from build123d import *

# Parameters (mm, degrees)
BOSS_EXTRUDE1_DEPTH      = 170
SKETCH7_W                = 5
SKETCH7_H                = 142.5
BOSS_EXTRUDE2_DEPTH      = 130
SKETCH9_W                = 160
SKETCH9_H                = 130
CUT_EXTRUDE2_DEPTH       = 60
SKETCH10_W               = 165
SKETCH10_H               = 3.7
CUT_EXTRUDE3_DEPTH       = 137.5
SKETCH13_W               = 160
SKETCH13_H               = 6
CUT_EXTRUDE4_DEPTH       = 5
SKETCH15_W               = 20
SKETCH15_H               = 10
BOSS_EXTRUDE3_DEPTH      = 70
SKETCH16_W               = 25
SKETCH16_H               = 12.5
CUT_EXTRUDE5_DEPTH       = 5
M6_CLEARANCE_HOLE1_D     = 7
M6_CLEARANCE_HOLE1_DEPTH = 10
SKETCH26_W               = 30
SKETCH26_H               = 9.35
CUT_EXTRUDE6_DEPTH       = 68.2
SKETCH27_W               = 30
SKETCH27_H               = 9.35
CUT_EXTRUDE8_DEPTH       = 68.2
CUT_EXTRUDE10_DEPTH      = 5
CUT_EXTRUDE11_DEPTH      = 5
SKETCH30_W               = 30
SKETCH30_H               = 9.35
CUT_EXTRUDE12_DEPTH      = 68.2
CUT_EXTRUDE14_DEPTH      = 54.5
FILLET1_R                = 2


with BuildPart() as part:
    # Sketch1 → Boss-Extrude1 (new body)
    with BuildSketch(Plane(origin=(0, 0, 0), x_dir=(0, 0, -1), z_dir=(1, 0, 0))):
        Polygon((90, 142.5), (90, 0), (85, 0), (85, 137.5), (-45, 137.5), (-45, 0), (-50, 0), (-50, 142.5), align=None)
    extrude(amount=BOSS_EXTRUDE1_DEPTH)

    # Sketch7 → Boss-Extrude2 (add)
    with BuildSketch(Plane(origin=(0, 0, 45), x_dir=(-1, 0, 0), z_dir=(0, 0, -1))):
        with Locations((-167.5, 71.25)):
            Rectangle(SKETCH7_W, SKETCH7_H)
        with Locations((-2.5, 71.25)):
            Rectangle(SKETCH7_W, SKETCH7_H)
    extrude(amount=BOSS_EXTRUDE2_DEPTH)

    # Sketch9 → Cut-Extrude2 (cut)
    with BuildSketch(Plane(origin=(0, 142.5, 0), x_dir=(1, 0, 0), z_dir=(0, 1, 0))):
        with Locations((85, 20)):
            Rectangle(SKETCH9_W, SKETCH9_H)
    extrude(amount=-CUT_EXTRUDE2_DEPTH, mode=Mode.SUBTRACT)

    # Sketch10 → Cut-Extrude3 (cut)
    with BuildSketch(Plane(origin=(80, 0, -90), x_dir=(1, 0, 0), z_dir=(0, 0, 1))):
        with Locations((5, 137.65)):
            Rectangle(SKETCH10_W, SKETCH10_H)
    extrude(amount=CUT_EXTRUDE3_DEPTH, mode=Mode.SUBTRACT)

    # Sketch13 → Cut-Extrude4 (cut)
    with BuildSketch(Plane(origin=(80, 0, -90), x_dir=(1, 0, 0), z_dir=(0, 0, 1))):
        with Locations((5, 139.5)):
            Rectangle(SKETCH13_W, SKETCH13_H)
    extrude(amount=CUT_EXTRUDE4_DEPTH, mode=Mode.SUBTRACT)

    # Sketch15 → Boss-Extrude3 (add, symmetric)
    with BuildSketch(Plane.XY.offset(-20)):
        with Locations((-10, 5)):
            Rectangle(SKETCH15_W, SKETCH15_H)
        with Locations((180, 5)):
            Rectangle(SKETCH15_W, SKETCH15_H)
    extrude(amount=BOSS_EXTRUDE3_DEPTH, both=True)

    # Sketch16 → Cut-Extrude5 (cut)
    with BuildSketch(Plane.XY.offset(50)):
        with Locations((35, 115)):
            Rectangle(SKETCH16_W, SKETCH16_H)
        with Locations((135, 115)):
            Rectangle(SKETCH16_W, SKETCH16_H)
    cut_extrude5 = extrude(amount=-CUT_EXTRUDE5_DEPTH, mode=Mode.SUBTRACT)

    # M6 Clearance Hole1
    with Locations(Plane(origin=(0, 10, 0), x_dir=(1, 0, 0), z_dir=(0, 1, 0))):
        with Locations((-10, -15), (-10, 55), (180, 55), (180, -15)):
            Hole(M6_CLEARANCE_HOLE1_D / 2, depth=M6_CLEARANCE_HOLE1_DEPTH)

    # Mirror2: Cut-Extrude5 across plane
    add(cut_extrude5.mirror(Plane.XY.offset(-20)), mode=Mode.SUBTRACT)

    # Sketch26 → Cut-Extrude6 (cut, symmetric)
    with BuildSketch(Plane.XY.offset(-20)):
        with Locations((135, 128)):
            Rectangle(SKETCH26_W, SKETCH26_H)
        with Locations((35, 128)):
            Rectangle(SKETCH26_W, SKETCH26_H)
    extrude(amount=CUT_EXTRUDE6_DEPTH, both=True, mode=Mode.SUBTRACT)

    # Sketch27 → Cut-Extrude8 (cut)
    with BuildSketch(Plane.XY.offset(-20)):
        with Locations((85, 21.8)):
            Rectangle(SKETCH27_W, SKETCH27_H)
    extrude(amount=CUT_EXTRUDE8_DEPTH, mode=Mode.SUBTRACT)

    # Sketch28 → Cut-Extrude10 (cut)
    with BuildSketch(Plane(origin=(0, 0, 50), x_dir=(-1, 0, 0), z_dir=(0, 0, -1))):
        with BuildLine():
            Line((-72.5, 0), (-72.5, 13))
            ThreePointArc((-72.5, 13), (-73.085786438, 14.414213562), (-74.5, 15))
            Line((-74.5, 15), (-95.5, 15))
            ThreePointArc((-95.5, 15), (-96.914213562, 14.414213562), (-97.5, 13))
            Line((-97.5, 13), (-97.5, 0))
            Line((-97.5, 0), (-72.5, 0))
        make_face()
    extrude(amount=CUT_EXTRUDE10_DEPTH, mode=Mode.SUBTRACT)

    # Sketch29 → Cut-Extrude11 (cut)
    with BuildSketch(Plane.XY.offset(-90)):
        with BuildLine():
            Line((95.5, 52.5), (74.5, 52.5))
            ThreePointArc((74.5, 52.5), (73.085786438, 53.085786438), (72.5, 54.5))
            Line((72.5, 54.5), (72.5, 68))
            ThreePointArc((72.5, 68), (73.085786438, 69.414213562), (74.5, 70))
            Line((74.5, 70), (95.5, 70))
            ThreePointArc((95.5, 70), (96.914213562, 69.414213562), (97.5, 68))
            Line((97.5, 68), (97.5, 54.5))
            ThreePointArc((97.5, 54.5), (96.914213562, 53.085786438), (95.5, 52.5))
        make_face()
    extrude(amount=CUT_EXTRUDE11_DEPTH, mode=Mode.SUBTRACT)

    # Sketch30 → Cut-Extrude12 (cut)
    with BuildSketch(Plane.XY.offset(-20)):
        with Locations((85, 76.8)):
            Rectangle(SKETCH30_W, SKETCH30_H)
    extrude(amount=-CUT_EXTRUDE12_DEPTH, mode=Mode.SUBTRACT)

    # Sketch31 → Cut-Extrude14 (cut)
    with BuildSketch(Plane(origin=(0, 0, 0), x_dir=(1, 0, 0), z_dir=(0, 1, 0))):
        Polygon((97.5, 86.25), (100.5, 86.25), (100.5, 88.75), (97.5, 88.75), (97.5, 90), (72.5, 90), (72.5, 88.75), (69.5, 88.75), (69.5, 86.25), (72.5, 86.25), (72.5, 85), (97.5, 85), align=None)
    extrude(amount=CUT_EXTRUDE14_DEPTH, mode=Mode.SUBTRACT)

    # Fillet1
    fillet1_edges = [part.edges().sort_by_distance(p)[0] for p in [
        (0, 76.25, 50),
        (0, 142.5, -20),
        (0, 76.25, -90),
        (-10, 10, -90),
        (0, 10, -20),
        (-20, 5, -90),
        (-20, 10, -20),
        (-10, 10, 50),
        (-20, 5, 50),
        (190, 5, -90),
        (180, 10, -90),
        (190, 10, -20),
        (170, 10, -20),
        (190, 5, 50),
        (180, 10, 50),
        (85, 142.5, 50),
        (170, 76.25, -90),
        (170, 142.5, -20),
        (170, 76.25, 50),
    ]]
    fillet(fillet1_edges, radius=FILLET1_R)


solid = part.part
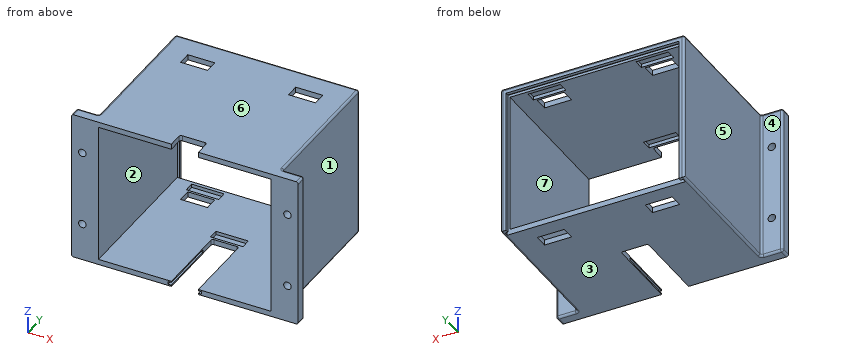
The model under review builds one solid part; all positions refer to its coordinate system, in mm. Face numbers are marked on the shaded views. A direction names the side the tool comes from. Round coordinates to 2 decimals unless told otherwise and drop trailing zeros. Write each loop counter-clockwise with the first axis right and the second up, starting at its lowest first coordinate (ties: lowest second). Pieces come first, ordered by that corner, then holes. Notation, with made-up numbers: (-20.5, 51) -> (-10.5, 51) arc R19 ccw to (-10.5, 59) -> close; hole circle Ø1 at (-25, 53.25). An arc over 180 degrees is marked (long way). Answer as a JSON object with one key per item and string values.
1. We need section B-B on z = -81. State the section outline as (x, y) points, and give its area (3 significant figures).
Results found:
{"outline": "(-20, 0) -> (5, 0) -> (5, 135.8) -> (2.5, 135.8) -> (2.5, 139.5) -> (5, 139.5) -> (5, 142.5) -> (2, 142.5) arc R2 ccw to (0, 140.5) -> (0, 12) arc R2 cw to (-2, 10) -> (-18, 10) arc R2 ccw to (-20, 8) -> close; (165, 0) -> (190, 0) -> (190, 8) arc R2 ccw to (188, 10) -> (172, 10) arc R2 cw to (170, 12) -> (170, 140.5) arc R2 ccw to (168, 142.5) -> (165, 142.5) -> (165, 139.5) -> (167.5, 139.5) -> (167.5, 135.8) -> (165, 135.8) -> close", "area": "1,800 mm^2"}
2. We need section A-A on x = 180. State the section outline as (y, z) points, and give its area (3 significant figures).
Results found:
{"outline": "(0, -90) -> (8, -90) arc R2 ccw to (10, -88) -> (10, -58.5) -> (0, -58.5) -> close; (0, -51.5) -> (10, -51.5) -> (10, 11.5) -> (0, 11.5) -> close; (0, 18.5) -> (10, 18.5) -> (10, 48) arc R2 ccw to (8, 50) -> (0, 50) -> close", "area": "1,260 mm^2"}
3. We need section D-D on y = 130. State the section outline as (x, z) points.
Results found:
{"outline": "(0, -88) arc R2 ccw to (2, -90) -> (168, -90) arc R2 ccw to (170, -88) -> (170, 48) arc R2 ccw to (168, 50) -> (2, 50) arc R2 ccw to (0, 48) -> close; hole (5, -85) -> (20, -85) -> (20, -88.2) -> (50, -88.2) -> (50, -85) -> (120, -85) -> (120, -88.2) -> (150, -88.2) -> (150, -85) -> (165, -85) -> (165, 45) -> (150, 45) -> (150, 48.2) -> (120, 48.2) -> (120, 45) -> (50, 45) -> (50, 48.2) -> (20, 48.2) -> (20, 45) -> (5, 45) -> close"}
4. To check wall thickness, follow line 1 along X through (y, z) = (4, -55); line 2 along Z through (x, y) = (-10, 7.25); line 3 along X through (y, z) = (42, 14). State the ranges of each line that lie inside material, in increasing order.
Results found:
{"line 1": "x = -20 to -13.5, -6.5 to 5, 165 to 176.5, 183.5 to 190", "line 2": "z = -90 to -58.5, -51.5 to 11.5, 18.5 to 50", "line 3": "x = 0 to 5, 165 to 170"}
5. The part is to be moulded in two halves that separate along X. For the marked faces 5, 6 and 7, say which applies: pulls with the +X half, pulls with the -X half, needs draft (parallel to the pull), parting line crosses it, or undercut.
Results found:
{"face 5": "pulls with the -X half", "face 6": "needs draft", "face 7": "undercut"}
6. Machinability: for the marked faces 1, 2, 3 and 4, which of the approach directions +Z, -Z, +X, -X, +Y, -Y give a long, thin tool a straight path to every point of the face, cutting with its end or side? Answer none if there is none.
Results found:
{"face 1": "+Z, -Z, +X, +Y", "face 2": "+Y, -Y", "face 3": "-Z, +X, -X, +Y, -Y", "face 4": "+Z, -Z, -X, +Y"}
7. Clearance check with flat-ended pins moving along their axes: pin 1 (0.8 mm diameter, centred on y = 23.5, z = -87, fed in from -X); pin 2 (1.6 mm diameter, centred on x = 140, z = -86.5, fed in from +Y); pin 3 (1 mm diameter, centred on x = 87, z = -86, fed in from -Y). State where each tip first meets the part, or that it passes through.
Results found:
{"pin 1": "stops at x = 0", "pin 2": "stops at y = 135.8", "pin 3": "stops at y = 70"}
8. We need section C-C on x = 62.5. State the section outline as (y, z) points, and give its area (3 significant figures).
Results found:
{"outline": "(0, -90) -> (135.8, -90) -> (135.8, -85) -> (0, -85) -> close; (0, 45) -> (135.8, 45) -> (135.8, 47.5) -> (139.5, 47.5) -> (139.5, 45) -> (142.5, 45) -> (142.5, 48) arc R2 ccw to (140.5, 50) -> (0, 50) -> close", "area": "1,380 mm^2"}
